from build123d import *

# Parameters (mm, degrees)
F0_W     = 180.17289
F0_H     = 124.226056
F1_DEPTH = 25.4
F2_R     = 9.959401
F2_R_2   = 10.991396
F3_DEPTH = 25.4
F4_R     = 50.24432
F5_DEPTH = 90.17
F6_W     = 106.479473
F6_H     = 50.532631
F7_DEPTH = 14.986


with BuildPart() as f1:
    # F0 (on Front) → F1 (new body)
    with BuildSketch(Plane.XZ):
        Rectangle(F0_W, F0_H)
    extrude(amount=F1_DEPTH)

    # F2 (on face) → F3 (join)
    with BuildSketch(Plane(origin=(-90.086445, 0, 0), x_dir=(0, -1, 0), z_dir=(-1, 0, 0))):
        with Locations((13.798693, 43.003704)):
            Circle(F2_R)
        with Locations((13.422888, -24.505027)):
            Circle(F2_R_2)
    extrude(amount=F3_DEPTH)

    # F4 (on face) → F5 (join)
    with BuildSketch(Plane(origin=(0, 0, 0), x_dir=(-1, 0, 0), z_dir=(0, 1, 0))):
        with Locations((0, -3.158289)):
            Circle(F4_R)
    extrude(amount=F5_DEPTH)

    # F6 (on face) → F7 (join)
    with BuildSketch(Plane.XZ.offset(25.4)):
        with Locations((61.143819, 40.756974)):
            Rectangle(F6_W, F6_H)
    extrude(amount=F7_DEPTH)


solid = f1.part
Build history of the part. All positions in model axes, mm. A direction names the side the tool comes from. Round coordinates to 2 decimals unless told otherwise and drop trailing zeros. Order: outer loops, then holes, each group sorted by start corner. A loop starts at its lowest first (then second) coordinate and runs counter-clockwise, first axis right, second up. Notation, with made-up numbers: M 16.25,65 L 51.25,65 A26 ccw 51.25,92 Z; hole C 12,54.25 d6. An arc over 180 degrees is marked long. Use CSV: the item, a comma, the result in double quotes. Start each with the question number.
(1) Mould opens along Z. For faces 1 (the face through (60, -33, 66.023)), 2 (the face through (7.904, -33, 40)), 3 (the face through (-102.61, -12.5, 52.88)) say: +Z half, -Z half, draft (parallel to the pull), parting line (faces both ways), or undercut.
(2) Drill centre lines: probe 1 along X at (y, z) = (-9.5, -34.5); probe 2 along Y at (x, z) = (-28.5, -41); probe 3 along Z at (x, y) = (32.5, -32.5). Where is each one in solid material? Low to high.
(3) Cut at D-D on z = -21.5. List the corners of the cut face in (x, y).
(4) Cut at B-B on z = 7.5. List the corners of the cut face in (x, y).
(5) Cut at A-A on x = 0. List the corners of the cut face in (y, z).
(6) Cut at C-C on y = 63.5. List the corners of the cut face in (x, z), then the cut area to 3 significant figures.
(7) Flat gauge pins, fed straight in: P1, Ø4, axis at y = -7, z = -19, coming from the +X side; P2, Ø8, axis at x = 45.5, y = 31, coming from the +Z side; P3, Ø3, axis at x = -18, z = 49.5, coming from the -Y side. Where does each tip first touch, or does it go through?
(8) Tool access for faces 4 (the face through (-102.609, -11.04, -35.235)), 5 (the face through (90.086, -13, -1)), 6 (the face through (-41, 0, 28)), 7 (the face through (60, -33, 15.491)): list every direction of +Z, -Z, +X, -X, +Y, -Y with a clear straight run to the whole face (end or side of a thin tool).
Findings:
1,face 1,"+Z half"
1,face 2,"draft"
1,face 3,"undercut"
2,probe 1,"x = -115.49 to 90.09"
2,probe 2,"y = -25.4 to 90.17"
2,probe 3,"z = 15.49 to 66.02"
3,outline,"M -115.49,-24 L -90.09,-24 L -90.09,-25.4 L 90.09,-25.4 L 90.09,0 L 46.78,0 L 46.78,90.17 L -46.78,90.17 L -46.78,0 L -90.09,0 L -90.09,-2.85 L -115.49,-2.85 Z"
4,outline,"M -90.09,-25.4 L 90.09,-25.4 L 90.09,0 L 49.1,0 L 49.1,90.17 L -49.1,90.17 L -49.1,0 L -90.09,0 Z"
5,outline,"M -25.4,-62.11 L 0,-62.11 L 0,-53.4 L 90.17,-53.4 L 90.17,47.09 L 0,47.09 L 0,62.11 L -25.4,62.11 Z"
6,outline,"C 0,-3.16 d100.49"
6,area,"7,930 mm^2"
7,P1,"stops at x = 90.09"
7,P2,"stops at z = 25.17"
7,P3,"stops at y = -25.4"
8,face 4,"-X"
8,face 5,"+Z, -Z, +X, +Y"
8,face 6,"+Y"
8,face 7,"-Z, +X, -X, -Y"
